Autodesk Fusion 360 part; units mm, degrees
sketch "Sketch1" plane through (0, 0, 0) normal (0, 1, 0) x (1, 0, 0)
  line L0 (30, 30) -> (30, -30)
  line L1 (30, -30) -> (-30, -30)
  line L2 (-30, -30) -> (-30, 30)
  line L3 (-30, 30) -> (30, -30) construction
  line L4 (30, 30) -> (-30, -30) construction
  line L5 (10, 30) -> (10, 50)
  line L6 (10, 50) -> (-10, 50)
  line L7 (-10, 50) -> (-10, 30)
  line L8 (-30, 30) -> (-10, 30)
  line L9 (10, 30) -> (30, 30)
  circle A0 centre (0, 43) radius 2.6
  line L10 (-30, 0) -> (30, 0) construction
  circle A1 centre (0, 21.5) radius 2.6
  circle A2 centre (-23, 21.5) radius 2.6
  circle A3 centre (23, 21.5) radius 2.6
  circle A4 centre (-10.75, 21.5) radius 1.25
  circle A5 centre (10.75, 21.5) radius 1.25
  circle A6 centre (-23, 0) radius 2.6
  circle A7 centre (-10.75, 0) radius 1.25
  circle A8 centre (0, 0) radius 2.6
  circle A9 centre (10.75, 0) radius 1.25
  circle A10 centre (23, 0) radius 2.6
  circle A11 centre (-23, -21.5) radius 2.6
  circle A12 centre (-10.75, -21.5) radius 1.25
  circle A13 centre (10.75, -21.5) radius 1.25
  circle A14 centre (23, -21.5) radius 2.6
  line L11 (-2.6, -21) -> (-2.6, -22)
  arc A15 (-2.6, -22) -> (2.6, -22) centre (0, -22) ccw
  line L12 (2.6, -22) -> (2.6, -21)
  arc A16 (2.6, -21) -> (-2.6, -21) centre (0, -21) ccw
  point P0 (0, -21.5)
  dimension "d4" = 60
  dimension "d5" = 60
  dimension "d7" = 20
  dimension "d8" = 20
  dimension "d9" = 5.2
  dimension "d10" = 7
  dimension "d11" = 5.2
  dimension "d12" = 21.5
  dimension "d13" = 5.2
  dimension "d14" = 5.2
  dimension "d15" = 23
  dimension "d16" = 23
  dimension "d17" = 2.5
  dimension "d18" = 2.5
  dimension "d19" = 10.75
  dimension "d20" = 10.75
  dimension "d24" = 21.5
  dimension "d25" = 0
  dimension "d28" = 5.2
  dimension "d29" = 0.5
extrude "Extrude1" add sketch "Sketch1" along normal blind 6
chamfer "Chamfer1" distance 6 angle 45 4 edges at (30, 3, 30) (30, 3, -30) (-30, 3, 30) (-30, 3, -30)
fillet "Fillet1" radius 3 2 edges at (10, 3, -50) (-10, 3, -50)
fillet "Fillet2" radius 3 2 edges at (10, 3, -30) (-10, 3, -30)
equation "larger_hole_radii = 2.6 mm"
equation "small_hole_Radii = 1.25 mm"
equation "base_sqaure_dim = 60 mm"
equation "d4 = base_sqaure_dim"
equation "d5 = base_sqaure_dim"
equation "square_extension = 20 mm"
equation "d7 = square_extension"
equation "d8 = square_extension"
equation "d9 = larger_hole_radii * 2"
equation "d11 = larger_hole_radii * 2"
equation "d13 = 2 * larger_hole_radii"
equation "d14 = 2 * larger_hole_radii"
equation "d17 = small_hole_Radii * 2"
equation "d18 = small_hole_Radii * 2"
equation "dist_between_Rows = 21.50 mm"
equation "slot_height = 5.20 mm"
equation "slot_width = 0.50 mm"
equation "d28 = slot_height"
equation "d29 = slot_width"
equation "ext = 6.0 mm"
equation "d31 = ext"
equation "d33 = ext"
equation "fillet_top = 3 mm"
equation "d36 = fillet_top"
equation "d38 = fillet_top"
The listing builds one solid part. Answer for the finished solid, in the listing's coordinates (mm). A direction names the side the tool comes from. Coordinates: 2 decimals unless noted, no trailing zeros. Loops run counter-clockwise (first coordinate to the right, second up) from the corner with the lowest first, then second, coordinate; pieces in that order, holes last. Notation, with made-up numbers: (-20, 24) - (27, 24) arc R16 ccw to (27, 48) - close; hole circle Ø8 at (75.25, 66.25). An arc over 180 degrees is marked (long way). Write item = value, one per line.
1) Each of these flat-tipped pins is pushed along its axis until it touches: P1, Ø3, axis at x = -23, z = 21.5, coming from the +Y side; P2, Ø2, axis at y = 4, z = -24.5, coming from the -X side; P3, Ø3, axis at y = 2, z = -38.5, coming from the -X side. Where does it stop, or does it pass through?
Responses:
P1 = through
P2 = -30
P3 = -10
2) Section D-D (x = -16.5) is taken. Determine the outline of the cut face in (y, z).
Responses:
outline = (0, -30) - (6, -30) - (6, 30) - (0, 30) - close
3) Find the intervals of material crossed by line 1 along X through (y, z) = (2.3, -21.5); line 2 along Z through (x, y) = (0, 3.9); line 3 along X through (y, z) = (0.3, 22), in increasing order.
Responses:
line_1 = -30 to -25.6, -20.4 to -12, -9.5 to -2.6, 2.6 to 9.5, 12 to 20.4, 25.6 to 30
line_2 = -50 to -45.6, -40.4 to -24.1, -18.9 to -2.6, 2.6 to 18.4, 24.6 to 30
line_3 = -30 to -25.55, -20.45 to -11.9, -9.6 to -2.6, 2.6 to 9.6, 11.9 to 20.45, 25.55 to 30
4) Section A-A (z = -21.5) is taken. Determine the outline of the cut face in (x, y).
Responses:
outline = (-30, 0) - (-25.6, 0) - (-25.6, 6) - (-30, 6) - close; (-20.4, 0) - (-12, 0) - (-12, 6) - (-20.4, 6) - close; (-9.5, 0) - (-2.6, 0) - (-2.6, 6) - (-9.5, 6) - close; (2.6, 0) - (9.5, 0) - (9.5, 6) - (2.6, 6) - close; (12, 0) - (20.4, 0) - (20.4, 6) - (12, 6) - close; (25.6, 0) - (30, 0) - (30, 6) - (25.6, 6) - close
5) Section B-B (z = -43) is taken. Determine the outline of the cut face in (x, y), plus the area to 3 significant figures.
Responses:
outline = (-10, 0) - (-2.6, 0) - (-2.6, 6) - (-10, 6) - close; (2.6, 0) - (10, 0) - (10, 6) - (2.6, 6) - close
area = 88.8 mm^2
6) Which of the six approach directions +Z, -Z, +X, -X, +Y, -Y give full straight-line access (tool end or side, diameter ignored) to faces 1 (the face through (0.1, 3, 24.6)), 2 (the face through (10, 3, -40)), 3 (the face through (-10, 3, -40)), 4 (the face through (-27, 3, 27)), 5 (the face through (0, 0, -11))?
Responses:
face_1 = +Y, -Y
face_2 = -Z, +X, +Y, -Y
face_3 = -Z, -X, +Y, -Y
face_4 = +Z, -X, +Y, -Y
face_5 = +Z, -Z, +X, -X, -Y
7) Section C-C (x = 11) is taken. Determine the outline of the cut face in (y, z).
Responses:
outline = (0, -30.76) - (6, -30.76) - (6, -22.72) - (0, -22.72) - close; (0, -20.28) - (6, -20.28) - (6, -1.22) - (0, -1.22) - close; (0, 1.22) - (6, 1.22) - (6, 20.28) - (0, 20.28) - close; (0, 22.72) - (6, 22.72) - (6, 30) - (0, 30) - close
